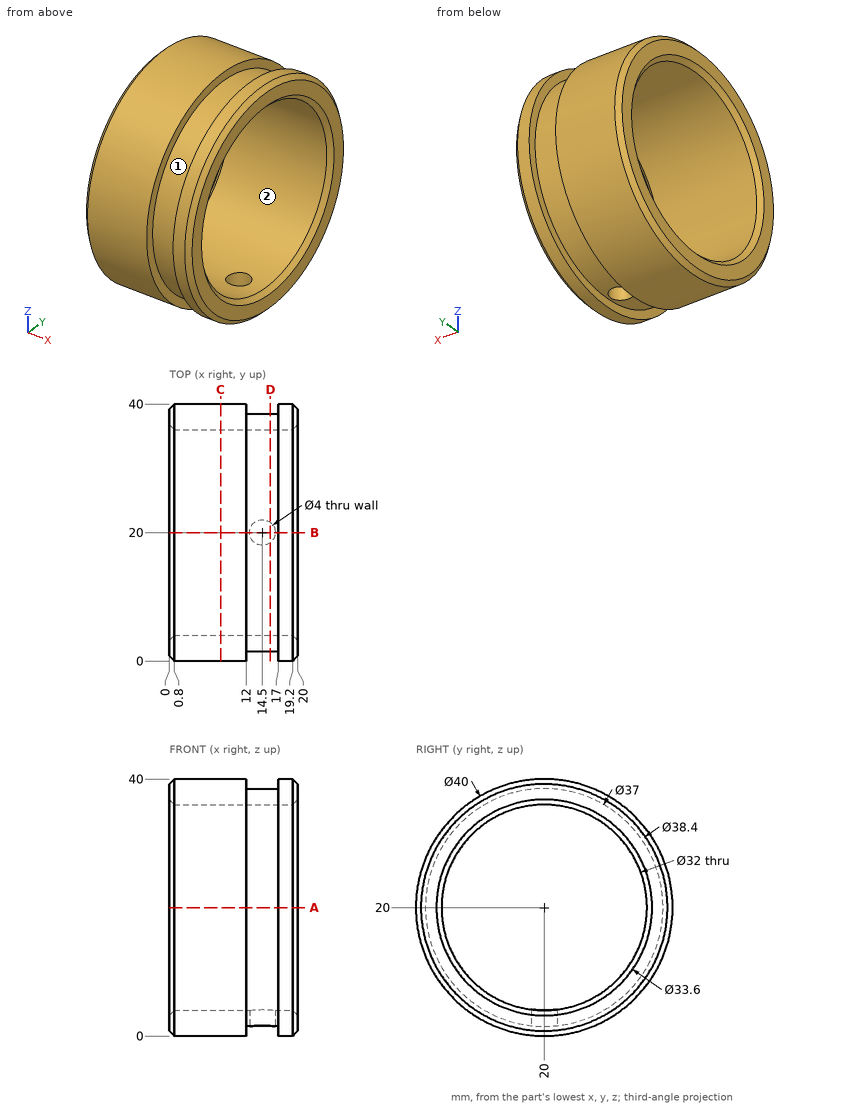
The drawing under review shows one solid part. Ordinate dimensions are in mm from its lowest x, y, z. Round coordinates to 2 decimals unless told otherwise and drop trailing zeros. Loops run counter-clockwise (first coordinate to the right, second up) from the corner with the lowest first, then second, coordinate; pieces in that order, holes last. Notation, with made-up numbers: (89, 5.5) - (130, 5.5) arc R30 ccw to (130, 39.5) - close; hole circle Ø8 at (38, 76.5). An arc over 180 degrees is marked (long way). Put each result on its own line as item: value. Start each with the question number.
1. For probe 1 along X at (y, z) = (38.5, 16.5); probe 2 along Z at (x, y) = (9.25, 20); probe 3 along X at (y, z) = (20, 2.2), list the stretches that pass through material, from the lowest coordinate up. Write a range as [from, to].
2. Consider section B-B on y = 20. State the section outline as (x, z) points, plus the area to 3 significant figures.
3. Insertion check: P1, Ø6, axis at x = 3.5, z = 30.5, coming from the -Y side; P2, Ø12, axis at y = 15.5, z = 13.5, coming from the +X side; P3, Ø1, axis at x = 2.5, y = 27, coming from the +Z side; P4, Ø6, axis at x = 10.5, y = 35, coming from the -Z side. Each pin has a flat end and moves straight along its axis. Give the tip position at first contact, or say it passes through.
4. Consider section D-D on x = 15.75. State the section outline as (y, z) points.
5. Mouldability with a two-part tool opening along Y and no side actions: class the marked faces 1 and 2 as +Y half, -Y half, draft (parallel to the pull), parting line (faces both ways), or undercut.
6. Consider section A-A on z = 20. State the section outline as (x, y) points, plus the area to 3 significant figures.
7. Consider section C-C on x = 8. State the section outline as (y, z) points, plus the area to 3 significant figures.
Result sheet:
1. probe 1: [0, 12], [17, 20]
1. probe 2: [0, 4], [36, 40]
1. probe 3: [0, 12.5], [16.5, 20]
2. outline: (0, 0.8) - (0.8, 0) - (12, 0) - (12, 1.5) - (12.5, 1.5) - (12.5, 4) - (0.8, 4) - (0, 3.2) - close; (0, 36.8) - (0.8, 36) - (19.2, 36) - (20, 36.8) - (20, 39.2) - (19.2, 40) - (17, 40) - (17, 38.5) - (12, 38.5) - (12, 40) - (0.8, 40) - (0, 39.2) - close; (16.5, 1.5) - (17, 1.5) - (17, 0) - (19.2, 0) - (20, 0.8) - (20, 3.2) - (19.2, 4) - (16.5, 4) - close
2. area: 132 mm^2
3. P1: y = 1.46
3. P2: through
3. P3: z = 38.91
3. P4: z = 4
4. outline: (18.44, 1.57) - (18.44, 4.08) arc R16 cw (long way) to (21.56, 4.08) - (21.56, 1.57) arc R18.5 ccw (long way) to start
5. face 1: parting line
5. face 2: undercut
6. outline: (0, 0.8) - (0.8, 0) - (12, 0) - (12, 1.5) - (17, 1.5) - (17, 0) - (19.2, 0) - (20, 0.8) - (20, 3.2) - (19.2, 4) - (0.8, 4) - (0, 3.2) - close; (0, 36.8) - (0.8, 36) - (19.2, 36) - (20, 36.8) - (20, 39.2) - (19.2, 40) - (17, 40) - (17, 38.5) - (12, 38.5) - (12, 40) - (0.8, 40) - (0, 39.2) - close
6. area: 142 mm^2
7. outline: circle Ø40 at (20, 20); hole circle Ø32 at (20, 20)
7. area: 452 mm^2
